Autodesk Inventor part; units mm, degrees
ref_plane "YZ Plane" through (0, 0, 0) normal (1, 0, 0) x (0, 1, 0)
ref_plane "XZ Plane" through (0, 0, 0) normal (0, 1, 0) x (-1, 0, 0)
ref_plane "XY Plane" through (0, 0, 0) normal (0, 0, 1) x (1, 0, 0)
sketch "Эскиз1" plane through (0, 0, 0) normal (0, 0, 1) x (1, 0, 0)
  circle A0 centre (0, 0) radius 75
  circle A1 centre (0, 0) radius 70
  line L0 (-75, 0) -> (75, 0)
  point P0 (70, 0)
  point P1 (-70, 0)
  dimension "d0" = 150
  dimension "d1" = 140
extrude "Выдавливание1" add sketch "Эскиз1" along normal blind 110 contours L0 A1 A0 picked at (0, 71.5073)
sketch "Эскиз2" plane through (0, 0, 0) normal (0, 1, 0) x (-1, 0, 0)
  line L0 (-75, 0) -> (75, 0)
  line L1 (75, 0) -> (75, 110)
  line L2 (-75, 110) -> (75, 110)
  line L3 (-75, 0) -> (-75, 110)
  circle A0 centre (0, 55) radius 5
  point P0 (0, 0)
  dimension "d4" = 10
extrude "Выдавливание2" cut sketch "Эскиз2" along normal blind 110 contours A0
properties part number "Под шатун" material "Бронза, литейная"
Work out the finished part from the listing and answer in its coordinate system (mm). Coordinates: 2 decimals unless noted, no trailing zeros. Loops run counter-clockwise (first coordinate to the right, second up) from the corner with the lowest first, then second, coordinate; pieces in that order, holes last.
1) Section A-A (x = 0) is taken. Give the vertices of the cut face in (y, z).
Results:
outline: (70, 0) - (75, 0) - (75, 50) - (70, 50) - close; (70, 60) - (75, 60) - (75, 110) - (70, 110) - close
2) Section D-D (x = 47) is taken. Give the vertices of the cut face in (y, z), plus the area to 3 significant figures.
Results:
outline: (51.87, 0) - (58.45, 0) - (58.45, 110) - (51.87, 110) - close
area: 723 mm2
3) For a pull along X with two mould halves and no side action, classify faces 1 (the cylindrical face through (-1.65, 74.98, 42.01)), 2 (the cylindrical face through (0.651, 72.374, 50.043)), 3 (the flat face through (72, 0, 54)) as +X half, -X half, draft (parallel to the pull), parting line (faces both ways), or undercut.
Results:
face 1: parting line
face 2: undercut
face 3: draft
4) Flat-ended cylindrical pins translate along their axes: pin 1 (8 mm diameter, centred on x = 0, z = 55, fed in from -Y); pin 2 (1.5 mm diameter, centred on x = -13.5, z = 20, fed in from +Y); pin 3 (8 mm diameter, centred on y = 23, z = 74, fed in from -X); pin 4 (12 mm diameter, centred on x = -32, z = 33, fed in from +Y). Find the tip coordinate at first contact, or state that the pin passes through.
Results:
pin 1: passes through
pin 2: stops at y = 73.91
pin 3: stops at x = -72.55
pin 4: stops at y = 70.35
5) Section C-C (z = 40.5) is taken. Give the vertices of the cut face in (x, y).
Results:
outline: (-75, 0) - (-70, 0) arc R70 cw to (70, 0) - (75, 0) arc R75 ccw to start
6) Section B-B (y = 67) is taken. Give the vertices of the cut face in (x, z), plus the area to 3 significant figures.
Results:
outline: (-33.7, 0) - (-20.27, 0) - (-20.27, 110) - (-33.7, 110) - close; (20.27, 0) - (33.7, 0) - (33.7, 110) - (20.27, 110) - close
area: 2,950 mm2
7) Consider probe 1 along Z at (x, y) = (0, 73); probe 2 along X at (y, z) = (61.5, 99); probe 3 along X at (y, z) = (9, 43.5). Determine where each line is inside the solid, lowest interval first.
Results:
probe 1: z = 0 to 50, 60 to 110
probe 2: x = -42.93 to -33.43, 33.43 to 42.93
probe 3: x = -74.46 to -69.42, 69.42 to 74.46
